Part model, mm, in its own coordinate system. Round coordinates to 2 decimals unless told otherwise and drop trailing zeros. Loops run counter-clockwise (first coordinate to the right, second up) from the corner with the lowest first, then second, coordinate; pieces in that order, holes last.
from build123d import *

# Parameters (mm, degrees)
SKETCH1_W                 = 201.168
SKETCH1_H                 = 201.168
BOSS_EXTRUDE1_DEPTH       = 1.5875
CUT_EXTRUDE1_REACH        = 144.256
SKETCH2_R                 = 17.4625
SKETCH2_R_2               = 16.5
F_1_4_CLEARANCE_HOLE1_D   = 6.7564
CHAMFER1_SIZE             = 6.35
CUT_EXTRUDE3_REACH        = 144.256
CUT_EXTRUDE4_REACH        = 144.256
CUT_EXTRUDE5_REACH        = 144.256
SKETCH7_W                 = 6.7564
SKETCH7_H                 = 14.478
SKETCH7_W_2               = 14.478
SKETCH7_H_2               = 6.7564
PORT_FOR_POWER_PLUG_REACH = 144.256
SKETCH8_R                 = 6.35


with BuildPart() as part:
    # Sketch1 → Boss-Extrude1 (new body)
    with BuildSketch(Plane.XY):
        Rectangle(SKETCH1_W, SKETCH1_H)
    extrude(amount=BOSS_EXTRUDE1_DEPTH)

    # Sketch2 → Cut-Extrude1 (cut, up to next)
    with BuildSketch(Plane.XY.offset(1.5875), mode=Mode.PRIVATE) as cut_extrude1_sk1:
        with Locations((-47.244, -40.5765)):
            Circle(SKETCH2_R)
    cut_extrude1_tool1 = extrude(cut_extrude1_sk1.sketch, amount=-CUT_EXTRUDE1_REACH, mode=Mode.PRIVATE) & part.part
    # Sketch2 → Cut-Extrude1 (cut, up to next)
    with BuildSketch(Plane.XY.offset(1.5875), mode=Mode.PRIVATE) as cut_extrude1_sk2:
        with Locations((39.4206, -52.284)):
            Circle(SKETCH2_R_2)
    cut_extrude1_tool2 = extrude(cut_extrude1_sk2.sketch, amount=-CUT_EXTRUDE1_REACH, mode=Mode.PRIVATE) & part.part
    add(cut_extrude1_tool1.solids().sort_by_distance((-47.244, -40.5765, 1.5875))[0], mode=Mode.SUBTRACT)
    add(cut_extrude1_tool2.solids().sort_by_distance((39.4206, -52.284, 1.5875))[0], mode=Mode.SUBTRACT)

    # 1/4 Clearance Hole1 (through all)
    with Locations(Plane.XY.offset(1.5875)):
        with Locations((-57.94375, 87.884), (57.94375, 87.884), (87.884, 0), (-87.884, 0), (-60.325, -87.884), (60.325, -87.884)):
            Hole(F_1_4_CLEARANCE_HOLE1_D / 2)

    # Chamfer1
    chamfer1_edges = [part.edges().sort_by_distance(p)[0] for p in [
        (100.584, -100.584, 0.79375),
        (-100.584, -100.584, 0.79375),
        (-100.584, 100.584, 0.79375),
        (100.584, 100.584, 0.79375),
    ]]
    chamfer(chamfer1_edges, length=CHAMFER1_SIZE)

    # Sketch5 → Cut-Extrude3 (cut, up to next)
    with BuildSketch(Plane(origin=(0, 0, 0), x_dir=(-1, 0, 0), z_dir=(0, 0, -1)), mode=Mode.PRIVATE) as cut_extrude3_sk1:
        with BuildLine():
            Line((29.7815, -40.5765), (29.7815, -71.0565))
            Line((29.7815, -71.0565), (64.7065, -71.0565))
            Line((64.7065, -71.0565), (64.7065, -40.5765))
            ThreePointArc((64.7065, -40.5765), (47.244, -58.039), (29.7815, -40.5765))
        make_face()
    cut_extrude3_tool1 = extrude(cut_extrude3_sk1.sketch, amount=-CUT_EXTRUDE3_REACH, mode=Mode.PRIVATE) & part.part
    add(cut_extrude3_tool1.solids().sort_by_distance((-47.244, -62.220952, 0))[0], mode=Mode.SUBTRACT)

    # Sketch6 → Cut-Extrude4 (cut, up to next)
    with BuildSketch(Plane(origin=(0, 0, 0), x_dir=(-1, 0, 0), z_dir=(0, 0, -1)), mode=Mode.PRIVATE) as cut_extrude4_sk1:
        with BuildLine():
            Line((-50.165, 49.768115066), (-50.165, 51.308))
            ThreePointArc((-50.165, 51.308), (-50.8, 51.943), (-51.435, 51.308))
            Line((-51.435, 51.308), (-51.435, 49.768115066))
            ThreePointArc((-51.435, 49.768115066), (-50.8, 24.384), (-50.165, 49.768115066))
        make_face()
    cut_extrude4_tool1 = extrude(cut_extrude4_sk1.sketch, amount=-CUT_EXTRUDE4_REACH, mode=Mode.PRIVATE) & part.part
    # Sketch6 → Cut-Extrude4 (cut, up to next)
    with BuildSketch(Plane(origin=(0, 0, 0), x_dir=(-1, 0, 0), z_dir=(0, 0, -1)), mode=Mode.PRIVATE) as cut_extrude4_sk2:
        with BuildLine():
            Line((51.435, 49.768115066), (51.435, 51.308))
            ThreePointArc((51.435, 51.308), (50.8, 51.943), (50.165, 51.308))
            Line((50.165, 51.308), (50.165, 49.768115066))
            ThreePointArc((50.165, 49.768115066), (50.8, 24.384), (51.435, 49.768115066))
        make_face()
    cut_extrude4_tool2 = extrude(cut_extrude4_sk2.sketch, amount=-CUT_EXTRUDE4_REACH, mode=Mode.PRIVATE) & part.part
    add(cut_extrude4_tool1.solids().sort_by_distance((50.8, 37.153354, 0))[0], mode=Mode.SUBTRACT)
    add(cut_extrude4_tool2.solids().sort_by_distance((-50.8, 37.153354, 0))[0], mode=Mode.SUBTRACT)

    # Sketch7 → Cut-Extrude5 (cut, up to next)
    with BuildSketch(Plane(origin=(0, 0, 0), x_dir=(-1, 0, 0), z_dir=(0, 0, -1)), mode=Mode.PRIVATE) as cut_extrude5_sk1:
        with Locations((-57.94375, 95.123)):
            Rectangle(SKETCH7_W, SKETCH7_H)
    cut_extrude5_tool1 = extrude(cut_extrude5_sk1.sketch, amount=-CUT_EXTRUDE5_REACH, mode=Mode.PRIVATE) & part.part
    # Sketch7 → Cut-Extrude5 (cut, up to next)
    with BuildSketch(Plane(origin=(0, 0, 0), x_dir=(-1, 0, 0), z_dir=(0, 0, -1)), mode=Mode.PRIVATE) as cut_extrude5_sk2:
        with Locations((57.94375, 95.123)):
            Rectangle(SKETCH7_W, SKETCH7_H)
    cut_extrude5_tool2 = extrude(cut_extrude5_sk2.sketch, amount=-CUT_EXTRUDE5_REACH, mode=Mode.PRIVATE) & part.part
    # Sketch7 → Cut-Extrude5 (cut, up to next)
    with BuildSketch(Plane(origin=(0, 0, 0), x_dir=(-1, 0, 0), z_dir=(0, 0, -1)), mode=Mode.PRIVATE) as cut_extrude5_sk3:
        with Locations((95.123, 0)):
            Rectangle(SKETCH7_W_2, SKETCH7_H_2)
    cut_extrude5_tool3 = extrude(cut_extrude5_sk3.sketch, amount=-CUT_EXTRUDE5_REACH, mode=Mode.PRIVATE) & part.part
    # Sketch7 → Cut-Extrude5 (cut, up to next)
    with BuildSketch(Plane(origin=(0, 0, 0), x_dir=(-1, 0, 0), z_dir=(0, 0, -1)), mode=Mode.PRIVATE) as cut_extrude5_sk4:
        with Locations((60.325, -95.123)):
            Rectangle(SKETCH7_W, SKETCH7_H)
    cut_extrude5_tool4 = extrude(cut_extrude5_sk4.sketch, amount=-CUT_EXTRUDE5_REACH, mode=Mode.PRIVATE) & part.part
    # Sketch7 → Cut-Extrude5 (cut, up to next)
    with BuildSketch(Plane(origin=(0, 0, 0), x_dir=(-1, 0, 0), z_dir=(0, 0, -1)), mode=Mode.PRIVATE) as cut_extrude5_sk5:
        with Locations((-60.325, -95.123)):
            Rectangle(SKETCH7_W, SKETCH7_H)
    cut_extrude5_tool5 = extrude(cut_extrude5_sk5.sketch, amount=-CUT_EXTRUDE5_REACH, mode=Mode.PRIVATE) & part.part
    # Sketch7 → Cut-Extrude5 (cut, up to next)
    with BuildSketch(Plane(origin=(0, 0, 0), x_dir=(-1, 0, 0), z_dir=(0, 0, -1)), mode=Mode.PRIVATE) as cut_extrude5_sk6:
        with Locations((-95.123, 0)):
            Rectangle(SKETCH7_W_2, SKETCH7_H_2)
    cut_extrude5_tool6 = extrude(cut_extrude5_sk6.sketch, amount=-CUT_EXTRUDE5_REACH, mode=Mode.PRIVATE) & part.part
    add(cut_extrude5_tool1.solids().sort_by_distance((57.94375, 95.123, 0))[0], mode=Mode.SUBTRACT)
    add(cut_extrude5_tool2.solids().sort_by_distance((-57.94375, 95.123, 0))[0], mode=Mode.SUBTRACT)
    add(cut_extrude5_tool3.solids().sort_by_distance((-95.123, 0, 0))[0], mode=Mode.SUBTRACT)
    add(cut_extrude5_tool4.solids().sort_by_distance((-60.325, -95.123, 0))[0], mode=Mode.SUBTRACT)
    add(cut_extrude5_tool5.solids().sort_by_distance((60.325, -95.123, 0))[0], mode=Mode.SUBTRACT)
    add(cut_extrude5_tool6.solids().sort_by_distance((95.123, 0, 0))[0], mode=Mode.SUBTRACT)

    # Sketch8 → PORT FOR POWER PLUG (cut, up to next)
    with BuildSketch(Plane(origin=(0, 0, 0), x_dir=(-1, 0, 0), z_dir=(0, 0, -1)), mode=Mode.PRIVATE) as port_for_power_plug_sk1:
        with Locations((-1.533105196, -45.535092969)):
            Circle(SKETCH8_R)
    port_for_power_plug_tool1 = extrude(port_for_power_plug_sk1.sketch, amount=-PORT_FOR_POWER_PLUG_REACH, mode=Mode.PRIVATE) & part.part
    add(port_for_power_plug_tool1.solids().sort_by_distance((1.533105, -45.535093, 0))[0], mode=Mode.SUBTRACT)


solid = part.part
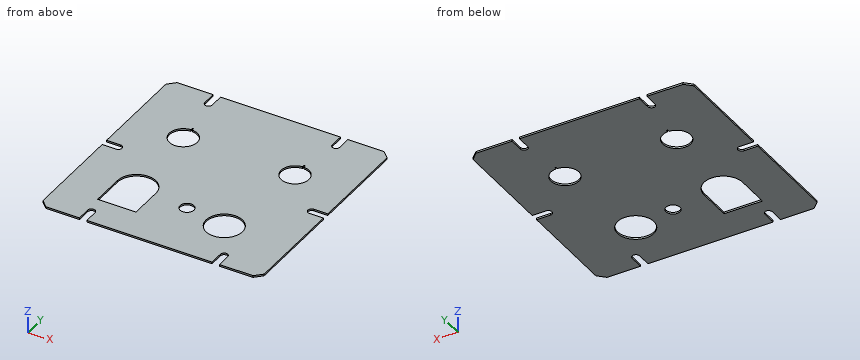
1) Slice it at A-A, the plane y = 28.5. Give the cut face in (x, z), then the cut area to 3 significant figures.
Values:
outline: (-100.58, 0) - (-60.16, 0) - (-60.16, 1.59) - (-100.58, 1.59) - close; (-41.44, 0) - (41.44, 0) - (41.44, 1.59) - (-41.44, 1.59) - close; (60.16, 0) - (100.58, 0) - (100.58, 1.59) - (60.16, 1.59) - close
area: 260 mm2
2) Wall check: line 1 along X through (y, z) = (-85, 0.9); line 2 along Y through (x, z) = (54, 0.2); line 3 along Y through (x, z) = (51, 0.9). Give the ranges that are in metal, low to high.
Values:
line 1: x = -100.58 to -62.08, -58.57 to 58.57, 62.08 to 100.58
line 2: y = -100.58 to -60.01, -44.56 to 24.79, 49.37 to 100.58
line 3: y = -100.58 to -64.04, -40.53 to 24.39, 51.91 to 100.58
3) Slice it at C-C, the plane y = 0. Give the cut face in (x, z).
Values:
outline: (-84.51, 0) - (84.51, 0) - (84.51, 1.59) - (-84.51, 1.59) - close
4) Slice it at B-B, the plane z = 0.7. Give the number of separate pieces and of enclosed holes in the cut face, then the cut area to 3 significant figures.
Values:
separate pieces: 1
enclosed holes: 5
area: 36,200 mm2
5) Drop a flat-ended pin along its axis: pin 1 Ø0.5 at (x, z) = (97, 0.5) entering from -Y. Give the stop position or say it passes through.
Values:
pin 1: stops at y = -98.07
